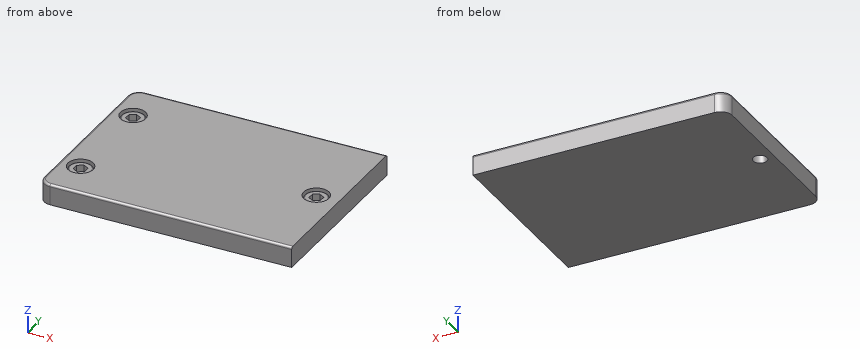
from build123d import *

# Parameters (mm, degrees)
BOSS_EXTRU_1_DEPTH               = 9
CONG_1_R                         = 1
ESQUISSE4_R                      = 5.5
ENL_V_MAT_EXTRU_1_DEPTH          = 7
ESQUISSE5_R                      = 5
BOSS_EXTRU_2_DEPTH               = 6
CONG_2_R                         = 0.5
ENL_V_MAT_EXTRU_2_DEPTH          = 4
R_P_TITION_LIN_AIRE1_COUNT       = 2
R_P_TITION_LIN_AIRE1_PITCH       = 44
CONG_2_OF_R_P_TITION_LIN_AIRE1_R = 0.5
ESQUISSE7_R                      = 5.5
ENL_V_MAT_EXTRU_3_DEPTH          = 7
ESQUISSE8_R                      = 5
BOSS_EXTRU_3_DEPTH               = 6
CONG_3_R                         = 0.5
ENL_V_MAT_EXTRU_4_DEPTH          = 5
ESQUISSE10_R                     = 3
ENL_V_MAT_EXTRU_5_DEPTH          = 5


with BuildPart() as part:
    # Esquisse1 → Boss.-Extru.1 (new body)
    with BuildSketch(Plane(origin=(0, 0, 0), x_dir=(-1, 0, 0), z_dir=(0, 0, 1))):
        with BuildLine():
            Line((0, 5), (0, 75))
            ThreePointArc((0, 75), (-1.464466094, 78.535533906), (-5, 80))
            Line((-5, 80), (-110, 80))
            Line((-110, 80), (-110, 0))
            Line((-110, 0), (-5, 0))
            ThreePointArc((-5, 0), (-1.464466094, 1.464466094), (0, 5))
        make_face()
    extrude(amount=BOSS_EXTRU_1_DEPTH)

    # Congé1
    cong_1_edges = [part.edges().sort_by_distance(p)[0] for p in [
        (1.464466094, -78.535533906, 9),
        (57.5, -80, 9),
        (57.5, 0, 9),
        (1.464466094, -1.464466094, 9),
        (0, -40, 9),
    ]]
    fillet(cong_1_edges, radius=CONG_1_R)

    # Esquisse4 → Enlèv. mat.-Extru.1 (cut)
    with BuildSketch(Plane.XY.offset(9)):
        with Locations((9, -18)):
            Circle(ESQUISSE4_R)
    enl_v_mat_extru_1 = extrude(amount=-ENL_V_MAT_EXTRU_1_DEPTH, mode=Mode.SUBTRACT)

    # Esquisse5 → Boss.-Extru.2 (add)
    with BuildSketch(Plane.XY.offset(2)):
        with Locations((9, -18)):
            Circle(ESQUISSE5_R)
    boss_extru_2 = extrude(amount=BOSS_EXTRU_2_DEPTH)

    # Congé2
    cong_2_edges = [part.edges().sort_by_distance(p)[0] for p in [
        (4, -18, 8),
    ]]
    fillet(cong_2_edges, radius=CONG_2_R)

    # Esquisse6 → Enlèv. mat.-Extru.2 (cut)
    with BuildSketch(Plane.XY.offset(8)):
        Polygon((9, -15.113248654), (6.5, -16.556624327), (6.5, -19.443375673), (9, -20.886751346), (11.5, -19.443375673), (11.5, -16.556624327), align=None)
    enl_v_mat_extru_2 = extrude(amount=-ENL_V_MAT_EXTRU_2_DEPTH, mode=Mode.SUBTRACT)

    # Répétition linéaire1: Enlèv. mat.-Extru.1, Boss.-Extru.2, Enlèv. mat.-Extru.2 ×2
    with Locations(*[(0, -i * R_P_TITION_LIN_AIRE1_PITCH, 0) for i in range(1, R_P_TITION_LIN_AIRE1_COUNT)]):
        add(enl_v_mat_extru_1, mode=Mode.SUBTRACT)
        add(boss_extru_2)
        add(enl_v_mat_extru_2, mode=Mode.SUBTRACT)

    # Congé2 of Répétition linéaire1
    cong_2_of_r_p_tition_lin_aire1_edges = [part.edges().sort_by_distance(p)[0] for p in [
        (4, -62, 8),
    ]]
    fillet(cong_2_of_r_p_tition_lin_aire1_edges, radius=CONG_2_OF_R_P_TITION_LIN_AIRE1_R)

    # Esquisse7 → Enlèv. mat.-Extru.3 (cut)
    with BuildSketch(Plane.XY.offset(9)):
        with Locations((100, -40)):
            Circle(ESQUISSE7_R)
    extrude(amount=-ENL_V_MAT_EXTRU_3_DEPTH, mode=Mode.SUBTRACT)

    # Esquisse8 → Boss.-Extru.3 (add)
    with BuildSketch(Plane.XY.offset(2)):
        with Locations((100, -40)):
            Circle(ESQUISSE8_R)
    extrude(amount=BOSS_EXTRU_3_DEPTH)

    # Congé3
    cong_3_edges = [part.edges().sort_by_distance(p)[0] for p in [
        (95, -40, 8),
    ]]
    fillet(cong_3_edges, radius=CONG_3_R)

    # Esquisse9 → Enlèv. mat.-Extru.4 (cut)
    with BuildSketch(Plane.XY.offset(8)):
        Polygon((100, -37.113248654), (97.5, -38.556624327), (97.5, -41.443375673), (100, -42.886751346), (102.5, -41.443375673), (102.5, -38.556624327), align=None)
    extrude(amount=-ENL_V_MAT_EXTRU_4_DEPTH, mode=Mode.SUBTRACT)

    # Esquisse10 → Enlèv. mat.-Extru.5 (cut)
    with BuildSketch(Plane(origin=(0, 0, 0), x_dir=(-1, 0, 0), z_dir=(0, 0, -1))):
        with Locations((-6, -40)):
            Circle(ESQUISSE10_R)
    extrude(amount=-ENL_V_MAT_EXTRU_5_DEPTH, mode=Mode.SUBTRACT)


solid = part.part
Geometry check sheet. Reference: the model listing, model coordinates, mm. Give positions to 0.01 mm unless a question says otherwise; leave off trailing zeros. Order: outer loops, then holes, each group sorted by start corner. A loop starts at its lowest first (then second) coordinate and runs counter-clockwise, first axis right, second up.
1) Cross-section at A-A (y = -40). Record the boundary of the cut face in (x, z).
Results are:
outline: (0, 0) - (3, 0) - (3, 5) - (9, 5) - (9, 0) - (110, 0) - (110, 9) - (105.5, 9) - (105.5, 2) - (105, 2) - (105, 7.5) arc R0.5 ccw to (104.5, 8) - (102.5, 8) - (102.5, 3) - (97.5, 3) - (97.5, 8) - (95.5, 8) arc R0.5 ccw to (95, 7.5) - (95, 2) - (94.5, 2) - (94.5, 9) - (1, 9) arc R1 ccw to (0, 8) - close
2) Gauge pin test, flat ends, axial feed: pin 1 (4.5 mm diameter, centred on x = 98, y = -40, fed in from +Z); pin 2 (1.5 mm diameter, centred on x = 8, y = -17.5, fed in from +Z). Record the tip position at first contact, or that the pin passes through.
Results are:
pin 1: stops at z = 8
pin 2: stops at z = 4
3) Material ranges on probe 1 along Y at (x, z) = (100, 5.25); probe 2 along X at (y, z) = (-67, 8.5), recorded low to high.
Results are:
probe 1: y = -80 to -45.5, -45 to -42.89, -37.11 to -35, -34.5 to 0
probe 2: x = 0.13 to 6.71, 11.29 to 110
